```python
from build123d import *

# Parameters (mm, degrees)
SKETCH1_W           = 16.5
SKETCH1_H           = 13.5
BOSS_EXTRUDE1_DEPTH = 15.65
SKETCH2_W           = 6.4
SKETCH2_H           = 5.096586226
SKETCH2_H_2         = 1.7
SKETCH2_H_3         = 0.9
CUT_EXTRUDE1_DEPTH  = 10


with BuildPart() as part:
    # Sketch1 → Boss-Extrude1 (new body)
    with BuildSketch(Plane.XY):
        Rectangle(SKETCH1_W, SKETCH1_H)
    extrude(amount=BOSS_EXTRUDE1_DEPTH)

    # Sketch2 → Cut-Extrude1 (cut)
    with BuildSketch(Plane.XY):
        Polygon((6.25, -4.85), (6.25, 3.15), (3.2, 3.15), (3.2, -1.946586226), (-3.2, -1.946586226), (-3.2, 3.15), (-6.25, 3.15), (-6.25, -4.85), align=None)
        with Locations((0, 0.601706887)):
            Rectangle(SKETCH2_W, SKETCH2_H)
        with Locations((0, 4)):
            Rectangle(SKETCH2_W, SKETCH2_H_2)
        with Locations((0, 5.3)):
            Rectangle(SKETCH2_W, SKETCH2_H_3)
    extrude(amount=CUT_EXTRUDE1_DEPTH, mode=Mode.SUBTRACT)


solid = part.part
```
Model file for the job. Use its own axes, mm. A direction names the side the tool comes from. Coordinates: 2 decimals unless noted, no trailing zeros. Loops run counter-clockwise (first coordinate to the right, second up) from the corner with the lowest first, then second, coordinate; pieces in that order, holes last. Notation, with made-up numbers: (70.5, 84.5) -> (97.5, 84.5) arc R15 ccw to (97.5, 111.5) -> close; hole circle Ø10 at (82, 12). An arc over 180 degrees is marked (long way). Answer as a JSON object with one key per item and string values.
Q1. Pull direction Y, two halves, no side cores. Call faces 1 (the flat face through (3.2, 4, 5)), 2 (the flat face through (-8.25, 0, 8)), 3 (the flat face through (6.25, -1, 5)), 4 (the flat face through (0, -6.75, 8)): released by +Y, released by -Y, zero draft, split by the parting line, or undercut.
Report:
{"face 1": "undercut", "face 2": "zero draft", "face 3": "undercut", "face 4": "released by -Y"}
Q2. Cut at B-B (x = 0). List the corners of the cut face in (y, z).
Report:
{"outline": "(-6.75, 0) -> (-4.85, 0) -> (-4.85, 10) -> (5.75, 10) -> (5.75, 0) -> (6.75, 0) -> (6.75, 15.65) -> (-6.75, 15.65) -> close"}
Q3. Flat gauge pin, fed straight in: P1, Ø5, axis at x = 2.5, y = -1, coming from the -Z side. Where does the tip first touch, or does it go through?
Report:
{"P1": "stops at z = 10"}
Q4. Probe probe 1 along X at (y, z) = (-0.5, 2.25); probe 2 along Y at (x, z) = (3.75, 2); probe 3 along X at (y, z) = (4.25, 2.75). List the from-to ranges inside material, lowest first.
Report:
{"probe 1": "x = -8.25 to -6.25, 6.25 to 8.25", "probe 2": "y = -6.75 to -4.85, 3.15 to 6.75", "probe 3": "x = -8.25 to -3.2, 3.2 to 8.25"}
Q5. Cut at C-C (y = 4.75). List the corners of the cut face in (x, z), and give its area (3 significant figures).
Report:
{"outline": "(-8.25, 0) -> (-3.2, 0) -> (-3.2, 10) -> (3.2, 10) -> (3.2, 0) -> (8.25, 0) -> (8.25, 15.65) -> (-8.25, 15.65) -> close", "area": "194 mm2"}
Q6. 3-axis set-ups, long thin cutter, end or side, ignore diameter. For faces 5 (the flat face through (-4, 5, 0)), 6 (the flat face through (0, -4.85, 5)): which of +Z, -Z, +X, -X, +Y, -Y reach the whole face in a straight line?
Report:
{"face 5": "-Z, +X, -X, +Y, -Y", "face 6": "-Z"}
Q7. Cut at A-A (z = 1.75). List the corners of the cut face in (x, y).
Report:
{"outline": "(-8.25, -6.75) -> (8.25, -6.75) -> (8.25, 6.75) -> (-8.25, 6.75) -> close; hole (-6.25, -4.85) -> (6.25, -4.85) -> (6.25, 3.15) -> (3.2, 3.15) -> (3.2, 5.75) -> (-3.2, 5.75) -> (-3.2, 3.15) -> (-6.25, 3.15) -> close"}
